Check sheet for the modelled part. Datum: model origin and axes. Units: mm. Round coordinates to 2 decimals unless told otherwise and drop trailing zeros. Write each loop counter-clockwise with the first axis right and the second up, starting at its lowest first coordinate (ties: lowest second). Pieces come first, ordered by that corner, then holes. Notation, with made-up numbers: (22, -8.75) -> (48, -8.75) arc R11 cw to (48, 5.25) -> close; hole circle Ø9 at (72, 16). An arc over 180 degrees is marked (long way). One line per item, written item: value.
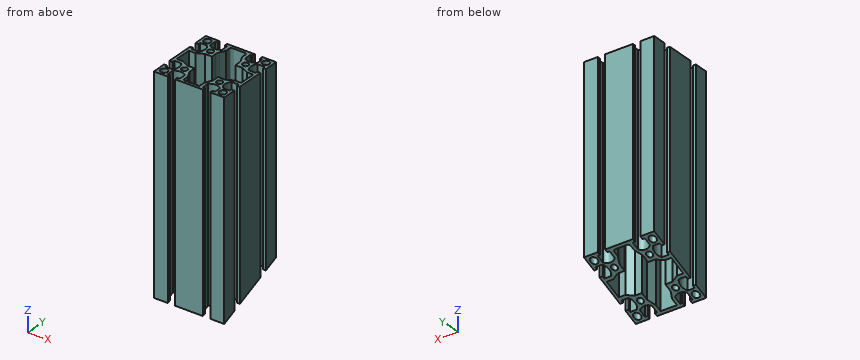
from build123d import *

# Parameters (mm, degrees)
F0_R          = 3
F0_R_2        = 2.5
F1_DEPTH      = 180
F2_R          = 2
F3_R          = 7
F6_DEPTH      = 30
F6_DEPTH_BACK = 30


# Not quite as in the source:
# - a feature names something its author has since deleted; it is built from what else it names


with BuildPart() as f1:
    # F0 (on Top) → F1 (new body)
    with BuildSketch(Plane.XY):
        with BuildLine():
            Line((18.15, -30), (30, -30))
            Line((30, -30), (30, -18.15))
            Line((30, -18.15), (27.5, -18.15))
            Line((27.5, -18.15), (27.5, -20.15))
            Line((27.5, -20.15), (21.5477069044, -20.15))
            ThreePointArc((21.5477069044, -20.15), (19.5, -15), (21.5477069044, -9.85))
            Line((21.5477069044, -9.85), (27.5, -9.85))
            Line((27.5, -9.85), (27.5, -11.85))
            Line((27.5, -11.85), (30, -11.85))
            Line((30, -11.85), (30, 11.85))
            Line((30, 11.85), (27.5, 11.85))
            Line((27.5, 11.85), (27.5, 9.85))
            Line((27.5, 9.85), (21.5477069044, 9.85))
            ThreePointArc((21.5477069044, 9.85), (19.5, 15), (21.5477069044, 20.15))
            Line((21.5477069044, 20.15), (27.5, 20.15))
            Line((27.5, 20.15), (27.5, 18.15))
            Line((27.5, 18.15), (30, 18.15))
            Line((30, 18.15), (30, 30))
            Line((30, 30), (18.15, 30))
            Line((18.15, 30), (18.15, 27.5))
            Line((18.15, 27.5), (20.15, 27.5))
            Line((20.15, 27.5), (20.15, 21.5477069044))
            ThreePointArc((20.15, 21.5477069044), (15, 19.5), (9.85, 21.5477069044))
            Line((9.85, 21.5477069044), (9.85, 27.5))
            Line((9.85, 27.5), (11.85, 27.5))
            Line((11.85, 27.5), (11.85, 30))
            Line((11.85, 30), (-11.85, 30))
            Line((-11.85, 30), (-11.85, 27.5))
            Line((-11.85, 27.5), (-9.85, 27.5))
            Line((-9.85, 27.5), (-9.85, 21.5477069044))
            ThreePointArc((-9.85, 21.5477069044), (-15, 19.5), (-20.15, 21.5477069044))
            Line((-20.15, 21.5477069044), (-20.15, 27.5))
            Line((-20.15, 27.5), (-18.15, 27.5))
            Line((-18.15, 27.5), (-18.15, 30))
            Line((-18.15, 30), (-30, 30))
            Line((-30, 30), (-30, 18.15))
            Line((-30, 18.15), (-27.5, 18.15))
            Line((-27.5, 18.15), (-27.5, 20.15))
            Line((-27.5, 20.15), (-21.5477069044, 20.15))
            ThreePointArc((-21.5477069044, 20.15), (-19.5, 15), (-21.5477069044, 9.85))
            Line((-21.5477069044, 9.85), (-27.5, 9.85))
            Line((-27.5, 9.85), (-27.5, 11.85))
            Line((-27.5, 11.85), (-30, 11.85))
            Line((-30, 11.85), (-30, -11.85))
            Line((-30, -11.85), (-27.5, -11.85))
            Line((-27.5, -11.85), (-27.5, -9.85))
            Line((-27.5, -9.85), (-21.5477069044, -9.85))
            ThreePointArc((-21.5477069044, -9.85), (-19.5, -15), (-21.5477069044, -20.15))
            Line((-21.5477069044, -20.15), (-27.5, -20.15))
            Line((-27.5, -20.15), (-27.5, -18.15))
            Line((-27.5, -18.15), (-30, -18.15))
            Line((-30, -18.15), (-30, -30))
            Line((-30, -30), (-18.15, -30))
            Line((-18.15, -30), (-18.15, -27.5))
            Line((-18.15, -27.5), (-20.15, -27.5))
            Line((-20.15, -27.5), (-20.15, -21.5477069044))
            ThreePointArc((-20.15, -21.5477069044), (-15, -19.5), (-9.85, -21.5477069044))
            Line((-9.85, -21.5477069044), (-9.85, -27.5))
            Line((-9.85, -27.5), (-11.85, -27.5))
            Line((-11.85, -27.5), (-11.85, -30))
            Line((-11.85, -30), (11.85, -30))
            Line((11.85, -30), (11.85, -27.5))
            Line((11.85, -27.5), (9.85, -27.5))
            Line((9.85, -27.5), (9.85, -21.5477069044))
            ThreePointArc((9.85, -21.5477069044), (15, -19.5), (20.15, -21.5477069044))
            Line((20.15, -21.5477069044), (20.15, -27.5))
            Line((20.15, -27.5), (18.15, -27.5))
            Line((18.15, -27.5), (18.15, -30))
        make_face()
        with Locations((-25, -25)):
            Circle(F0_R, mode=Mode.SUBTRACT)
        with Locations((-15, -15)):
            Circle(F0_R_2, mode=Mode.SUBTRACT)
        with Locations((25, -25)):
            Circle(F0_R, mode=Mode.SUBTRACT)
        with Locations((15, -15)):
            Circle(F0_R_2, mode=Mode.SUBTRACT)
        with Locations((-25, 25)):
            Circle(F0_R, mode=Mode.SUBTRACT)
        with Locations((-15, 15)):
            Circle(F0_R_2, mode=Mode.SUBTRACT)
        Polygon((-7, 22), (-7, 27.5), (0, 27.5), (7, 27.5), (7, 22), (10, 16), (10, 10), (16, 10), (22, 7), (27.5, 7), (27.5, 0), (27.5, -7), (22, -7), (16, -10), (10, -10), (10, -16), (7, -22), (7, -27.5), (0, -27.5), (-7, -27.5), (-7, -22), (-10, -16), (-10, -10), (-16, -10), (-22, -7), (-27.5, -7), (-27.5, 0), (-27.5, 7), (-22, 7), (-16, 10), (-10, 10), (-10, 16), align=None, mode=Mode.SUBTRACT)
        with Locations((15, 15)):
            Circle(F0_R_2, mode=Mode.SUBTRACT)
        with Locations((25, 25)):
            Circle(F0_R, mode=Mode.SUBTRACT)
    extrude(amount=F1_DEPTH)

    # F2
    f2_edges = [f1.edges().sort_by_distance(p)[0] for p in [
        (-7, 27.5, 90),
        (7, 27.5, 90),
    ]]
    fillet(f2_edges, radius=F2_R)

    # F3
    f3_edges = [f1.edges().sort_by_distance(p)[0] for p in [
        (-10, 16, 90),
        (10, 16, 90),
    ]]
    fillet(f3_edges, radius=F3_R)

    # F5 (on Right) → F6 (cut, two sides)
    with BuildSketch(Plane.YZ) as f6_sk:
        Polygon((189.0217391842, -31.0070544887), (145.9840988475, 72.8950005046), (-30, 0), (13.0376403367, -103.9020549933), align=None)
    extrude(amount=-F6_DEPTH, mode=Mode.SUBTRACT)
    extrude(f6_sk.sketch, amount=F6_DEPTH_BACK, mode=Mode.SUBTRACT)


solid = f1.part
Item 1: Sectioned sample at C-C (x = 25). Enter the section's corners in (y, z), then the cut area to 3 significant figures.
Result set:
outline: (-30, 0) -> (-28, 0.83) -> (-28, 180) -> (-30, 180) -> close; (-22, 3.31) -> (-20.15, 4.08) -> (-20.15, 180) -> (-22, 180) -> close; (-9.85, 8.35) -> (-7, 9.53) -> (-7, 180) -> (-9.85, 180) -> close; (7, 15.33) -> (9.85, 16.51) -> (9.85, 180) -> (7, 180) -> close; (20.15, 20.77) -> (22, 21.54) -> (22, 180) -> (20.15, 180) -> close; (28, 24.02) -> (30, 24.85) -> (30, 180) -> (28, 180) -> close
area: 2,250 mm^2
Item 2: Material ranges on line 1 along Y through (x, z) = (25, 98); line 2 along X through (y, z) = (-15, 66), recorded low to high.
Result set:
line 1: -30 to -28, -22 to -20.15, -9.85 to -7, 7 to 9.85, 20.15 to 22, 28 to 30
line 2: -19.5 to -17.5, -12.5 to -10, 10 to 12.5, 17.5 to 19.5
Item 3: Sectioned sample at A-A (x = -3). Enter the section's corners in (y, z), then the cut area to 3 significant figures.
Result set:
outline: (-30, 0) -> (-27.5, 1.04) -> (-27.5, 180) -> (-30, 180) -> close; (27.5, 23.82) -> (30, 24.85) -> (30, 180) -> (27.5, 180) -> close
area: 838 mm^2
Item 4: Sectioned sample at B-B (y = 2). Enter the section's corners in (x, z).
Result set:
outline: (-30, 13.25) -> (-27.5, 13.25) -> (-27.5, 180) -> (-30, 180) -> close; (27.5, 13.25) -> (30, 13.25) -> (30, 180) -> (27.5, 180) -> close
Item 5: Sectioned sample at D-D (z = 30.5). State how many separate pieces and enclosed holes the cut face has, then the cut area to 3 significant figures.
Result set:
separate pieces: 1
enclosed holes: 9
area: 1,080 mm^2
Item 6: Depth check by flat-ended pin: pin 1 (9.5 mm diameter, centred on x = -25, y = -25, fed in from -Z); pin 2 (8 mm diameter, centred on x = -19.5, y = -1.5, fed in from +Z); pin 3 (4 mm diameter, centred on x = -14, z = 161, fed in from -Y); pin 4 (8 mm diameter, centred on x = -7.5, y = 9.5, fed in from -Z). Enter the tip coordinate at first touch or a pass-through.
Result set:
pin 1: z = 0.1
pin 2: through
pin 3: y = -20.13
pin 4: z = 16.57
